Read the model definition and answer for the solid it produces. Units are mm, in the model's axes. A direction names the side the tool comes from. Coordinates: 2 decimals unless noted, no trailing zeros. Order: outer loops, then holes, each group sorted by start corner. A loop starts at its lowest first (then second) coordinate and runs counter-clockwise, first axis right, second up. Notation, with made-up numbers: M -22.5,70 L -14.5,70 A13 ccw -14.5,91 Z; hole C 66,44.5 d10. An arc over 180 degrees is marked long. Use a Markdown table: item, result. Add a question column.
1) For faces 4 (the face through (7, -1, 5)), 5 (the face through (-14, 16.7, 14)), 6 (the face through (-9, 33, 6)), 7 (the face through (-1, 5, 5)), determine the directions among +Z, -Z, +X, -X, +Y, -Y from which every point of the face is accessible in a straight line to the end or side of a thin tool.
2) Find the intervals of material crossed by probe 1 along Y at (x, z) = (-14, 2.75); probe 2 along Y at (x, z) = (-15.5, 7.75); probe 3 along Y at (x, z) = (-15.5, 13.5), in increasing order. Write a range as [from, to].
3) Find section A-A on x = -11. Write down the section's boundary in (y, z), plus the area to 4 significant figures.
4) Find section D-D on z = 8.5. Write down the section's boundary in (x, y), plus the area to 3 significant figures.
5) Each of these flat-tipped pins is pushed along its axis until it touches: pin 1 Ø1.9 at (x, y) = (-12.5, 15.5) entering from +Z; pin 2 Ø1.5 at (x, z) = (-14.5, 15) entering from -Y; pin 3 Ø1.5 at (x, z) = (-10.5, 17) entering from -Y. Where does it stop, or does it pass through?
6) Find section B-B on z = 11.5. Write down the section's boundary in (x, y), plus the area to 3 significant figures.
7) Find section C-C on y = 32.5. Write down the section's boundary in (x, z), plus the area to 3 significant figures.
8) The mould has two halves that part along Z. Classify faces 1 (the face through (-20, 17, 6)), 2 (the face through (-11, 34, 10)), 3 (the face through (-19.6, 17, 15.5)): released by +Z, released by -Z, zero draft, split by the parting line, or undercut.
from build123d import *

# Parameters (mm, degrees)
PAD_DEPTH       = 20.5
SKETCH003_W     = 34.5
SKETCH003_H     = 9
POCKET_DEPTH    = 10.5
POCKET001_DEPTH = 20
SKETCH018_W     = 13.6
SKETCH018_H     = 20.5
POCKET002_DEPTH = 10
SKETCH019_W     = 11
SKETCH019_H     = 10
POCKET003_DEPTH = 10.5
SKETCH020_W     = 6
SKETCH020_H     = 10
POCKET004_DEPTH = 10
SKETCH021_R     = 5.5
POCKET005_DEPTH = 1.7
SKETCH022_W     = 5
SKETCH022_H     = 5.5
POCKET006_DEPTH = 1.7
SKETCH023_R     = 5.5
POCKET007_DEPTH = 1.7
SKETCH024_W     = 5
SKETCH024_H     = 5.5
POCKET008_DEPTH = 1.7
SKETCH025_W     = 13.6
SKETCH025_H     = 5.500002
POCKET009_DEPTH = 1
SKETCH026_R     = 1
PAD001_DEPTH    = 1.5
FILLET_R        = 0.3
SKETCH027_R     = 1
PAD002_DEPTH    = 1.5
FILLET001_R     = 0.3


with BuildPart() as part:
    # Sketch → Pad (new body)
    with BuildSketch(Plane.XY):
        Polygon((13, 0), (13, -2.5), (14.5, -2.5), (14.5, -4), (5.5, -4), (5.5, -2.5), (7, -2.5), (7, 0), (-7, 0), (-7, -2.5), (-5.5, -2.5), (-5.5, -4), (-14.5, -4), (-14.5, -2.5), (-13, -2.5), (-13, 0), (-20, 0), (-20, 35), (-9, 35), (-9, 5), (13, 5), align=None)
    extrude(amount=PAD_DEPTH)

    # Sketch003 (on Face23 of Pad) → Pocket (cut)
    with BuildSketch(Plane.XY.offset(20.5)):
        with Locations((-2.75, 0.5)):
            Rectangle(SKETCH003_W, SKETCH003_H)
    extrude(amount=-POCKET_DEPTH, mode=Mode.SUBTRACT)

    # Sketch001 (on Face18 of Pad) → Pocket001 (cut)
    with BuildSketch(Plane(origin=(0, 35, 0), x_dir=(-1, 0, 0), z_dir=(0, 1, 0))):
        with BuildLine():
            ThreePointArc((19, 15.500002), (13.999998, 20.5), (9, 15.499998))
            Line((9, 21.5), (9, 15.499998))
            Line((9, 21.5), (20, 21.5))
            Line((20, 21.5), (20, 15.500002))
            Line((19, 15.500002), (20, 15.500002))
        make_face()
    extrude(amount=-POCKET001_DEPTH, mode=Mode.SUBTRACT)

    # Sketch018 (on Face22 of Pocket001) → Pocket002 (cut)
    with BuildSketch(Plane.YZ.offset(-9)):
        with Locations((25, 10.25)):
            Rectangle(SKETCH018_W, SKETCH018_H)
    extrude(amount=-POCKET002_DEPTH, mode=Mode.SUBTRACT)

    # Sketch019 (on Face29 of Pocket002) → Pocket003 (cut)
    with BuildSketch(Plane.XY.offset(20.5)):
        with Locations((-14.5, 10)):
            Rectangle(SKETCH019_W, SKETCH019_H)
    extrude(amount=-POCKET003_DEPTH, mode=Mode.SUBTRACT)

    # Sketch020 (on Face28 of Pocket003) → Pocket004 (cut)
    with BuildSketch(Plane.XY.offset(10)):
        with Locations((-12, 10)):
            Rectangle(SKETCH020_W, SKETCH020_H)
    extrude(amount=-POCKET004_DEPTH, mode=Mode.SUBTRACT)

    # Sketch021 (on Face15 of Pocket004) → Pocket005 (cut)
    with BuildSketch(Plane(origin=(0, 35, 0), x_dir=(-1, 0, 0), z_dir=(0, 1, 0))):
        with Locations((14, 15.5)):
            Circle(SKETCH021_R)
    extrude(amount=-POCKET005_DEPTH, mode=Mode.SUBTRACT)

    # Sketch022 (on Face15 of Pocket005) → Pocket006 (cut)
    with BuildSketch(Plane(origin=(0, 35, 0), x_dir=(-1, 0, 0), z_dir=(0, 1, 0))):
        with Locations((11.5, 12.75)):
            Rectangle(SKETCH022_W, SKETCH022_H)
    extrude(amount=-POCKET006_DEPTH, mode=Mode.SUBTRACT)

    # Sketch023 (on Face32 of Pocket006) → Pocket007 (cut)
    with BuildSketch(Plane.XZ.offset(-15)):
        with Locations((-14, 15.5)):
            Circle(SKETCH023_R)
    extrude(amount=-POCKET007_DEPTH, mode=Mode.SUBTRACT)

    # Sketch024 (on Face33 of Pocket007) → Pocket008 (cut)
    with BuildSketch(Plane.XZ.offset(-15)):
        with Locations((-11.5, 12.75)):
            Rectangle(SKETCH024_W, SKETCH024_H)
    extrude(amount=-POCKET008_DEPTH, mode=Mode.SUBTRACT)

    # Sketch025 (on Face12 of Pocket008) → Pocket009 (cut)
    with BuildSketch(Plane.YZ.offset(-19)):
        with Locations((25, 12.750001)):
            Rectangle(SKETCH025_W, SKETCH025_H)
    extrude(amount=-POCKET009_DEPTH, mode=Mode.SUBTRACT)

    # Sketch026 (on Face51 of Pocket009) → Pad001 (join)
    with BuildSketch(Plane.XZ.offset(-16.7)):
        with Locations((-14, 15.5)):
            Circle(SKETCH026_R)
    extrude(amount=PAD001_DEPTH)

    # Fillet
    fillet_edges = [part.edges().sort_by_distance(p)[0] for p in [
        (-15, 15.2, 15.5),
    ]]
    fillet(fillet_edges, radius=FILLET_R)

    # Sketch027 (on Face55 of Fillet) → Pad002 (join)
    with BuildSketch(Plane(origin=(0, 33.3, 0), x_dir=(-1, 0, 0), z_dir=(0, 1, 0))):
        with Locations((14, 15.5)):
            Circle(SKETCH027_R)
    extrude(amount=PAD002_DEPTH)

    # Fillet001
    fillet001_edges = [part.edges().sort_by_distance(p)[0] for p in [
        (-13, 34.8, 15.5),
    ]]
    fillet(fillet001_edges, radius=FILLET001_R)


solid = part.part
Check result:
| question | item | result |
|---|---|---|
| 1 | face 4 | +Z, -Z |
| 1 | face 5 | -Y |
| 1 | face 6 | +Z, -Z, +X, +Y |
| 1 | face 7 | +Z, -Z, +X |
| 2 | probe 1 | y = [-4, -2.5], [0, 5], [15, 18.2], [31.8, 35] |
| 2 | probe 2 | y = [0, 18.2], [31.8, 35] |
| 2 | probe 3 | y = [16.7, 18.2], [31.8, 33.3] |
| 3 | outline | M -4,0 L 5,0 L 5,10 L -4,10 Z; M 15,0 L 18.2,0 L 18.2,19.5 L 16.7,19.5 L 16.7,10 L 15,10 Z; M 31.8,0 L 35,0 L 35,10 L 33.3,10 L 33.3,19.5 L 31.8,19.5 Z |
| 3 | area | 182.5 mm2 |
| 4 | outline | M -20,0 L -13,0 L -13,-2.5 L -14.5,-2.5 L -14.5,-4 L -5.5,-4 L -5.5,-2.5 L -7,-2.5 L -7,0 L 7,0 L 7,-2.5 L 5.5,-2.5 L 5.5,-4 L 14.5,-4 L 14.5,-2.5 L 13,-2.5 L 13,5 L -15,5 L -15,15 L -9,15 L -9,18.2 L -19,18.2 L -19,31.8 L -9,31.8 L -9,35 L -20,35 Z |
| 4 | area | 356 mm2 |
| 5 | pin 1 | stops at z = 16.34 |
| 5 | pin 2 | stops at y = 15.2 |
| 5 | pin 3 | stops at y = 16.7 |
| 6 | outline | M -20,15 L -17.77,15 L -17.77,16.7 L -9,16.7 L -9,18.2 L -20,18.2 Z; M -20,31.8 L -9,31.8 L -9,33.3 L -17.77,33.3 L -17.77,35 L -20,35 Z |
| 6 | area | 40.6 mm2 |
| 7 | outline | M -20,0 L -9,0 L -9,15.5 A5 ccw -19,15.5 L -20,15.5 Z |
| 7 | area | 210 mm2 |
| 8 | face 1 | zero draft |
| 8 | face 2 | undercut |
| 8 | face 3 | released by +Z |
